Geometry check sheet. Reference: the model listing, model coordinates, mm. A direction names the side the tool comes from. Round coordinates to 2 decimals unless told otherwise and drop trailing zeros. Order: outer loops, then holes, each group sorted by start corner. A loop starts at its lowest first (then second) coordinate and runs counter-clockwise, first axis right, second up. Notation, with made-up numbers: (34.25, 64.25) -> (51.25, 64.25) arc R11 ccw to (51.25, 77.25) -> close; hole circle Ø4 at (-15.75, 75). An arc over 180 degrees is marked (long way). Use a Markdown table: item, result. Add a question column.
Item 1: Set-up check for faces 5 (the flat face through (1, -13, -55)), 6 (the flat face through (-20, 28.45, -27)), 7 (the flat face through (1, 2, -65)), 8 (the flat face through (1, 9, 5)): record each of +Z, -Z, +X, -X, +Y, -Y from which the full face is reachable in a straight line by a thin tool's end or side.
Item 2: Sectioned sample at A-A, the plane y = -16. State how many separate pieces and enclosed holes the cut face has, and give its area (3 significant figures).
Item 3: Gauge pin test, flat ends, axial feed: pin 1 Ø4 at (x, y) = (-21, -9) entering from +Z; pin 2 Ø2 at (x, z) = (-32.5, -2) entering from -Y; pin 3 Ø22.5 at (x, y) = (-0.5, 11.5) entering from +Z; pin 4 Ø8 at (y, z) = (-0.5, -62) entering from -X. Record the tip position at first contact, or that the pin passes through.
Item 4: Sectioned sample at B-B, the plane z = 2.5. Record the cut outline in (x, y), and give its area (3 significant figures).
Item 5: Material ranges on probe 1 along X at (y, z) = (-16, -60.25); probe 2 along Z at (x, y) = (10.5, -12); probe 3 along Z at (x, y) = (19.5, 12), recorded low to high. Write a range as [from, to].
Item 6: Sectioned sample at D-D, the plane y = 20. Record the cut outline in (x, z).
Item 7: Mould release check, pull along X, two halves, no side actions. Record for faces 1 (the flat face through (-26, -3, -61)), 2 (the cylindrical face through (0.491, -13.706, 4.93)), 3 (the flat face through (2, 9, -60)), 4 (the cylindrical face through (-23.348, -8.897, -59.93)): pulls with the +X half, pulls with the -X half, needs draft (parallel to the pull), parting line crosses it, or undercut.
Autodesk Inventor part; units mm, degrees
ref_plane "Work Plane2" through (-91.43, -48.7723, -27.5) normal (0, 0, 1) x (1, 0, 0)
ref_plane "YZ Plane" through (0, 0, 0) normal (1, 0, 0) x (0, 1, 0)
ref_plane "XZ Plane" through (0, 0, 0) normal (0, 1, 0) x (-1, 0, 0)
ref_plane "Work Plane1" through (0, 0, -55) normal (0, 0, -1) x (1, 0, 0)
sketch "Sketch2" plane through (0, 0, -55) normal (0, 0, -1) x (1, 0, 0)
  circle A0 centre (23, 9) radius 2.35
  circle A1 centre (1, 9) radius 2.35
  circle A2 centre (-21, 9) radius 2.35
  circle A3 centre (-21, 16) radius 2.35
  circle A4 centre (1, 16) radius 2.35
  circle A5 centre (23, 16) radius 2.35
  circle A6 centre (-66, 12.5) radius 1.6
  circle A7 centre (63, 29.65) radius 1.6
  arc A8 (58.9857, 35) -> (49.7248, 32.4349) centre (58.9857, 17) ccw
  line L0 (33.2752, 22.5651) -> (49.7248, 32.4349)
  arc A9 (24.0143, 20) -> (33.2752, 22.5651) centre (24.0143, 38) ccw
  line L1 (-71, 20) -> (24.0143, 20)
  arc A10 (-71, 20) -> (-81, 10) centre (-71, 10) ccw
  line L2 (-81, 6.5495) -> (-81, 10)
  line L3 (-80.0877, 6.5495) -> (-81, 6.5495)
  line L4 (81, 6.5495) -> (-80.0877, 6.5495)
  line L5 (81, 20) -> (81, 6.5495)
  arc A11 (81, 20) -> (66, 35) centre (66, 20) ccw
  line L6 (58.9857, 35) -> (66, 35)
  line L7 (-21, 16) -> (-26, 16)
  line L8 (-21, 16) -> (-16, 16) construction
  line L9 (-26, 16) -> (-26, 20)
  line L10 (-26, 20) -> (29, 20)
  line L11 (29, 20) -> (29, 6.5495)
  line L12 (29, 6.5495) -> (-26, 6.5495)
  line L13 (-26, 6.5495) -> (-26, 20)
  point P0 (0, 0)
  dimension "d0" = 5
  dimension "d1" = 180
  dimension "d2" = 55
extrude "Extrusion1" add sketch "Sketch2" along normal blind 10 contours L9 L1 L10 L11 L4 L13
sketch "Sketch3" plane through (-26, -6.5495, -55) normal (0, 1, 0) x (1, 0, 0)
  line L0 (0, 0) -> (0, 10)
  line L1 (0, 10) -> (55, 10)
  line L2 (55, 10) -> (55, 5)
  line L3 (55, 5) -> (0, 5)
  line L4 (0, 5) -> (0, 10)
  point P0 (26, -55)
  dimension "d5" = 55
  dimension "d6" = 5
extrude "Extrusion2" add sketch "Sketch3" along normal blind 35
sketch "Sketch4" plane through (-26, -6.5495, -60) normal (0, 0, 1) x (1, 0, 0)
  line L0 (0, -13.4505) -> (0, 35)
  line L1 (0, 35) -> (55, 35)
  line L2 (55, 35) -> (55, 32)
  line L3 (55, 32) -> (0, 32)
  line L4 (0, 32) -> (0, 35)
  point P0 (26, 6.5495)
  dimension "d9" = 55
  dimension "d10" = 3
ref_plane "Work Plane2" through (-91.43, -48.7723, -27.5) normal (0, 0, 1) x (1, 0, 0)
extrude "Extrusion3" add sketch "Sketch4" along normal up to surface (32.5 mm away)
ref_plane "Work Plane3" through (-26, -6.5495, -27.5) normal (0, 0, 1) x (1, 0, 0)
mirror "Mirror1" about plane through (-26, -6.5495, -27.5) normal (0, 0, 1) of "Extrusion3", "Extrusion2", "Extrusion1"
ref_plane "Work Plane4" through (-26, 25.4505, -55) normal (0, 1, 0) x (1, 0, 0)
sketch "Sketch5" plane through (-26, 25.4505, -55) normal (0, 1, 0) x (1, 0, 0)
  line L0 (55, 5) -> (55, -60)
  line L1 (55, -27.5) -> (55, -77.5)
  line L2 (55, -27.5) -> (105, -27.5) construction
  line L3 (55, -77.5) -> (-45, -77.5)
  line L4 (-45, -77.5) -> (-45, 22.5)
  line L5 (-45, 22.5) -> (55, 22.5)
  line L6 (55, 22.5) -> (55, -77.5)
  point P0 (26, -55)
  dimension "d15" = 50
  dimension "d16" = 90
  dimension "d17" = 100
  dimension "d18" = 100
extrude "Extrusion4" add sketch "Sketch5" along normal blind 3
Found:
| question | item | result |
|---|---|---|
| 1 | face 5 | +X, -X, -Y |
| 1 | face 6 | +Z, -Z, +X, -X, +Y |
| 1 | face 7 | -Z, +X, -X, -Y |
| 1 | face 8 | +X, -X |
| 2 | separate pieces | 8 |
| 2 | enclosed holes | 0 |
| 2 | area | 818 mm2 |
| 3 | pin 1 | passes through |
| 3 | pin 2 | stops at y = 25.45 |
| 3 | pin 3 | stops at z = 10 |
| 3 | pin 4 | stops at x = -26 |
| 4 | outline | (-71, 25.45) -> (29, 25.45) -> (29, 28.45) -> (-71, 28.45) -> close; (-26, -20) -> (29, -20) -> (29, -6.55) -> (-26, -6.55) -> close; hole circle Ø4.7 at (-21, -16); hole circle Ø4.7 at (-21, -9); hole circle Ø4.7 at (1, -16); hole circle Ø4.7 at (1, -9); hole circle Ø4.7 at (23, -16); hole circle Ø4.7 at (23, -9) |
| 4 | area | 936 mm2 |
| 5 | probe 1 | x = [-26, -23.35], [-18.65, -1.35], [3.35, 20.65], [25.35, 29] |
| 5 | probe 2 | z = [-65, -55], [0, 10] |
| 5 | probe 3 | z = [-65, -60], [5, 10] |
| 6 | outline | (-26, -65) -> (29, -65) -> (29, -60) -> (-26, -60) -> close; (-26, 5) -> (29, 5) -> (29, 10) -> (-26, 10) -> close |
| 7 | face 1 | pulls with the -X half |
| 7 | face 2 | undercut |
| 7 | face 3 | needs draft |
| 7 | face 4 | undercut |
